Here's how the part is built. I have some questions about the finished solid (model axes, mm). Face numbers are marked on the shaded views. A direction names the side the tool comes from. Coordinates: 2 decimals unless noted, no trailing zeros. Write each loop counter-clockwise with the first axis right and the second up, starting at its lowest first coordinate (ties: lowest second). Pieces come first, ordered by that corner, then holes. Notation, with made-up numbers: M 45,79.5 L 65,79.5 A12 ccw 65,88.5 Z; hole C -31.75,23 d7. An arc over 180 degrees is marked long. Use one line per item in the form item = value. Start each with the question number.
1. I want a section at A-A, the plane z = 0. List the corners of the cut face in (x, y) for me (3 decimals), plus the area to 3 significant figures.
2. Thinking about a two-plate mould opening in Z: for the marked faces 3, 4, 5 and 6, which applies, released by +Z, released by -Z, zero draft, split by the parting line, or undercut?
3. I want a section at C-C, the plane y = 6.75. List the corners of the cut face in (x, z) for me, plus the area to 3 significant figures.
4. I want a section at B-B, the plane x = 0. List the corners of the cut face in (y, z) for me (3 decimals).
5. Please list where these lines run through material, in increasing order: line 1 along X through (y, z) = (5, 0); line 2 along Z through (x, y) = (2, 5.25). Write a range as [from, to].
6. I'm going to push flat-ended pins straight in: pin 1 Ø5.5 at (x, z) = (0, 0) entering from -Y; pin 2 Ø2 at (x, z) = (3.5, -5.5) entering from -Y. Where does each tip first touch, or does it pass through?
7. I want a section at D-D, the plane x = -4.25. Count the separate pieces of the cut face and the enclosed holes in it, plus the area to 3 significant figures.
8. On a 3-axis mill with a long thin cutter (end or side, diameter ignored), from which of +Z, -Z, +X, -X, +Y, -Y can I reach the whole of each face in a straight line? I mean the marked faces 1 and 2. Say none if no direction works.
from build123d import *

# Parameters (mm, degrees)
BOSS_EXTRUDE1_DEPTH = 8
FILLET2_R           = 1.4
FILLET3_R           = 0.7


with BuildPart() as part:
    # Sketch1 → Boss-Extrude1 (new body)
    with BuildSketch(Plane(origin=(0, 0, 0), x_dir=(1, 0, 0), z_dir=(0, 1, 0))):
        with BuildLine():
            Line((-8, 5.123475383), (-8, -5.123475383))
            ThreePointArc((-8, -5.123475383), (-6.717514421, -6.717514421), (-5.123475383, -8))
            Line((-5.123475383, -8), (5.123475383, -8))
            ThreePointArc((5.123475383, -8), (6.717514421, -6.717514421), (8, -5.123475383))
            Line((8, -5.123475383), (8, 5.123475383))
            ThreePointArc((8, 5.123475383), (6.717514421, 6.717514421), (5.123475383, 8))
            Line((5.123475383, 8), (-5.123475383, 8))
            ThreePointArc((-5.123475383, 8), (-6.717514421, 6.717514421), (-8, 5.123475383))
        make_face()
    extrude(amount=BOSS_EXTRUDE1_DEPTH)

    # Sketch2 → Cut-Revolve1 (revolve, cut)
    with BuildSketch(Plane.XY, mode=Mode.PRIVATE) as cut_revolve1_sk:
        Polygon((6.9, 8), (7.477350269, 7), (9.756701135, 7), (9.756701135, 8), align=None)
    revolve(cut_revolve1_sk.sketch.rotate(Axis((0, 0, 0), (0, 1, 0)), 90), axis=Axis((0, 0, 0), (0, 1, 0)), mode=Mode.SUBTRACT)

    # Sketch5 → M10x1.0 Tapped Hole1 (revolve, cut)
    with BuildSketch(Plane(origin=(0, 0, 0), x_dir=(0, 0, -1), z_dir=(1, 0, 0))):
        Polygon((0, 0), (0, 8), (5.125, 8), (4.5, 7.375), (4.5, 0.625), (5.125, 0), align=None)
    revolve(axis=Axis((0, -6.35, 0), (0, 1, 0)), mode=Mode.SUBTRACT)

    # M3 Tapped Hole1: read off the stored shape, not the designer's step
    # M3 Tapped Hole1 outline → M3 Tapped Hole1 (revolve, cut)
    with BuildSketch(Plane(origin=(0, 4.19513424, 0), x_dir=(0.7071067811865471, 0, -0.707106781186548), z_dir=(0, -1, 0))):
        Polygon((0, -9.500060785), (1.525060785, -9.500060785), (1.25, -9.225), (1.25, -4.322803032), (0, -4.322803032), align=None)
    revolve(axis=Axis((0, 4.19513424, 0), (0.707106781186548, 0, 0.7071067811865471)), mode=Mode.SUBTRACT)

    # Fillet2
    fillet2_edges = [part.edges().sort_by_distance(p)[0] for p in [
        (6.717514421, 0, 6.717514421),
        (-6.717514421, 0, 6.717514421),
        (-6.717514421, 0, -6.717514421),
        (6.717514421, 0, -6.717514421),
    ]]
    fillet(fillet2_edges, radius=FILLET2_R)

    # Fillet3
    # the kernel refuses this fillet: 0.7 mm, written as the material it takes off along each edge
    with BuildSketch(Plane(origin=(0, 7, 0), x_dir=(-0.3759346527851674, 0, 0.9266461767229688), z_dir=(0.9266461767229688, 0, 0.3759346527851674))) as fillet3_piece_1:
        with BuildLine():
            CenterArc((9.5 - FILLET3_R, FILLET3_R), FILLET3_R, 270, 90)
            Line((9.5, FILLET3_R), (9.5, 0))
            Line((9.5, 0), (9.5 - FILLET3_R, 0))
        make_face()
    revolve(axis=Axis((0, 7, 0), (0, -1, 0)), revolution_arc=45.835816267, mode=Mode.SUBTRACT)
    with BuildSketch(Plane(origin=(0, 7, 0), x_dir=(-0.9266461767229688, 0, -0.3759346527851675), z_dir=(-0.3759346527851675, 0, 0.9266461767229688))) as fillet3_piece_2:
        with BuildLine():
            CenterArc((9.5 - FILLET3_R, FILLET3_R), FILLET3_R, 270, 90)
            Line((9.5 - FILLET3_R, 0), (9.5, 0))
            Line((9.5, 0), (9.5, FILLET3_R))
        make_face()
    revolve(axis=Axis((0, 7, 0), (0, -1, 0)), revolution_arc=45.835816267, mode=Mode.SUBTRACT)
    with BuildSketch(Plane(origin=(0, 7, 0), x_dir=(0.3759346527851687, 0, -0.9266461767229682), z_dir=(-0.9266461767229682, 0, -0.3759346527851687))) as fillet3_piece_3:
        with BuildLine():
            CenterArc((9.5 - FILLET3_R, FILLET3_R), FILLET3_R, 270, 90)
            Line((9.5 - FILLET3_R, 0), (9.5, 0))
            Line((9.5, 0), (9.5, FILLET3_R))
        make_face()
    revolve(axis=Axis((0, 7, 0), (0, -1, 0)), revolution_arc=45.835816267, mode=Mode.SUBTRACT)
    with BuildSketch(Plane(origin=(0, 7, 0), x_dir=(0.9266461767229706, 0, 0.3759346527851629), z_dir=(0.3759346527851629, 0, -0.9266461767229706))) as fillet3_piece_4:
        with BuildLine():
            CenterArc((9.5 - FILLET3_R, FILLET3_R), FILLET3_R, 270, 90)
            Line((9.5, FILLET3_R), (9.5, 0))
            Line((9.5, 0), (9.5 - FILLET3_R, 0))
        make_face()
    revolve(axis=Axis((0, 7, 0), (0, -1, 0)), revolution_arc=45.835816267, mode=Mode.SUBTRACT)
    with BuildSketch(Plane(origin=(8, 0, 6.518857754), x_dir=(-1, 0, 0), z_dir=(0, 0, -1)), Plane(origin=(-6.518857754, 0, 8), x_dir=(0, 0, -1), z_dir=(1, 0, 0)), Plane(origin=(-8, 0, -6.518857754), x_dir=(1, 0, 0), z_dir=(0, 0, 1))) as fillet3_piece_5:
        with BuildLine():
            CenterArc((FILLET3_R, FILLET3_R), FILLET3_R, 180, 90)
            Line((0, FILLET3_R), (0, 0))
            Line((0, 0), (FILLET3_R, 0))
        make_face()
    extrude(amount=13.037715508, mode=Mode.SUBTRACT)
    with BuildSketch(Plane(origin=(6.518857754, 0, -8), x_dir=(0, 1, 0), z_dir=(-1, 0, 0))) as fillet3_piece_6:
        with BuildLine():
            CenterArc((FILLET3_R, -FILLET3_R), FILLET3_R, 90, 90)
            Line((0, -FILLET3_R), (0, 0))
            Line((0, 0), (FILLET3_R, 0))
        make_face()
    extrude(amount=13.037715508, mode=Mode.SUBTRACT)


solid = part.part
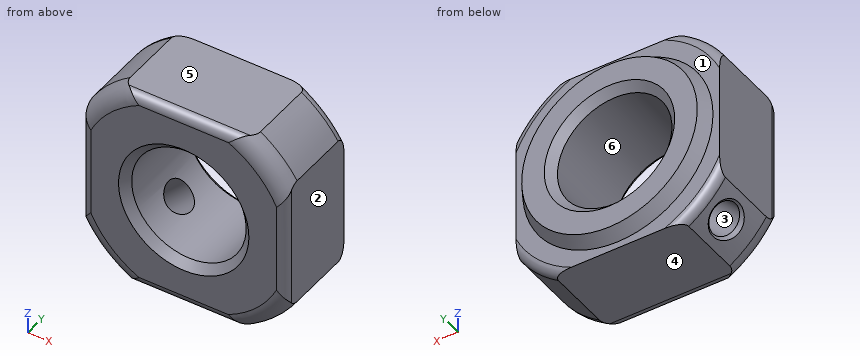
Answer list:
q1.outline = M -8,0.7 A0.7 ccw -7.3,0 L -5.125,0 L -4.5,0.625 L -4.5,7.375 L -5.125,8 L -6.9,8 L -7.477,7 L -8,7 Z; M 4.5,0.625 L 5.125,0 L 7.3,0 A0.7 ccw 8,0.7 L 8,7 L 7.477,7 L 6.9,8 L 5.125,8 L 4.5,7.375 Z
q1.area = 53.4 mm²
q2.face_3 = undercut
q2.face_4 = released by -Z
q2.face_5 = released by +Z
q2.face_6 = undercut
q3.outline = M -8,-4.81 A9.34 ccw -4.81,-8 L 4.81,-8 A9.34 ccw 8,-4.81 L 8,4.81 A9.34 ccw 4.81,8 L -4.81,8 A9.34 ccw -8,4.81 Z; hole C 0,0 d9
q3.area = 175 mm²
q4.outline = M 0,-7.3 A0.7 ccw 0.7,-8 L 7,-8 L 7,-7.477 L 8,-6.9 L 8,-5.125 L 7.375,-4.5 L 0.625,-4.5 L 0,-5.125 Z; M 0,5.125 L 0.625,4.5 L 7.375,4.5 L 8,5.125 L 8,6.9 L 7,7.477 L 7,8 L 0.7,8 A0.7 ccw 0,7.3 Z
q5.line_1 = [-8, -4.5], [4.5, 8]
q5.line_2 = [-8, -4.03], [4.03, 8]
q6.pin_1 = through
q6.pin_2 = 0
q7.separate_pieces = 2
q7.enclosed_holes = 1
q7.area = 90.8 mm²
q8.face_1 = +Y
q8.face_2 = +Z, -Z, +X, +Y, -Y
